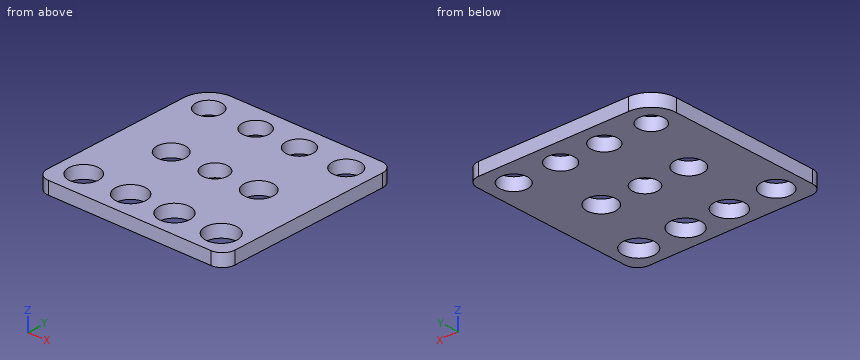
```python
from build123d import *

# Parameters (mm, degrees)
CROQUIS1_R              = 2.2
CROQUIS1_R_2            = 2.5
CROQUIS1_R_3            = 2.35
CROQUIS1_R_4            = 2.05
CROQUIS1_R_5            = 2.1
CROQUIS1_R_6            = 2.15
CROQUIS1_R_7            = 2.4
CROQUIS1_R_8            = 2.45
CROQUIS1_R_9            = 2.25
CROQUIS1_R_10           = 2.3
CROQUIS1_R_11           = 2
SALIENTE_EXTRUIR1_DEPTH = 2


with BuildPart() as part:
    # Croquis1 → Saliente-Extruir1 (new body)
    with BuildSketch(Plane.XY):
        with BuildLine():
            Line((-84.957262486, 47.717592446), (-60.957262486, 47.717592446))
            ThreePointArc((-60.957262486, 47.717592446), (-59.543048923, 47.131806009), (-58.957262486, 45.717592446))
            Line((-58.957262486, 45.717592446), (-58.957262486, 19.717592446))
            ThreePointArc((-58.957262486, 19.717592446), (-59.543048923, 18.303378884), (-60.957262486, 17.717592446))
            Line((-60.957262486, 17.717592446), (-86.957262486, 17.717592446))
            ThreePointArc((-86.957262486, 17.717592446), (-88.371476048, 18.303378884), (-88.957262486, 19.717592446))
            Line((-88.957262486, 19.717592446), (-88.957262486, 43.717592446))
            ThreePointArc((-88.957262486, 43.717592446), (-87.78568961, 46.546019571), (-84.957262486, 47.717592446))
        make_face()
        with Locations((-62.957262486, 43.717592446)):
            Circle(CROQUIS1_R, mode=Mode.SUBTRACT)
        with Locations((-62.957262486, 21.717592446)):
            Circle(CROQUIS1_R_2, mode=Mode.SUBTRACT)
        with Locations((-84.957262486, 21.717592446)):
            Circle(CROQUIS1_R_3, mode=Mode.SUBTRACT)
        with Locations((-84.957262486, 43.717592446)):
            Circle(CROQUIS1_R_4, mode=Mode.SUBTRACT)
        with Locations((-77.457263515, 43.721521604)):
            Circle(CROQUIS1_R_5, mode=Mode.SUBTRACT)
        with Locations((-70.457261138, 43.722088276)):
            Circle(CROQUIS1_R_6, mode=Mode.SUBTRACT)
        with Locations((-77.457263515, 21.721521604)):
            Circle(CROQUIS1_R_7, mode=Mode.SUBTRACT)
        with Locations((-70.457261138, 21.722088276)):
            Circle(CROQUIS1_R_8, mode=Mode.SUBTRACT)
        with Locations((-80.957262486, 32.717592446)):
            Circle(CROQUIS1_R_9, mode=Mode.SUBTRACT)
        with Locations((-66.957262486, 32.717592446)):
            Circle(CROQUIS1_R_10, mode=Mode.SUBTRACT)
        with Locations((-73.957262486, 32.717592446)):
            Circle(CROQUIS1_R_11, mode=Mode.SUBTRACT)
    extrude(amount=SALIENTE_EXTRUIR1_DEPTH)


solid = part.part
```
CAD build for the part. Positions are in the model's coordinates, mm. Round coordinates to 2 decimals unless told otherwise and drop trailing zeros. Write each loop counter-clockwise with the first axis right and the second up, starting at its lowest first coordinate (ties: lowest second). Pieces come first, ordered by that corner, then holes.
Item 1: Band-saw the part on C-C on z = 1.35. Give the number of separate pieces and of enclosed holes in the cut face, then the cut area to 3 significant figures.
Filled in:
separate pieces: 1
enclosed holes: 11
area: 718 mm2
Item 2: Band-saw the part on B-B on y = 22.5. Write the cut outline in (x, z).
Filled in:
outline: (-88.96, 0) - (-87.17, 0) - (-87.17, 2) - (-88.96, 2) - close; (-82.74, 0) - (-79.73, 0) - (-79.73, 2) - (-82.74, 2) - close; (-75.19, 0) - (-72.78, 0) - (-72.78, 2) - (-75.19, 2) - close; (-68.13, 0) - (-65.33, 0) - (-65.33, 2) - (-68.13, 2) - close; (-60.58, 0) - (-58.96, 0) - (-58.96, 2) - (-60.58, 2) - close
Item 3: Drop a flat-ended pin along its axis: pin 1 Ø3 at (x, y) = (-70.46, 21.72) entering from +Z. Give the stop position or say it passes through.
Filled in:
pin 1: passes through
Item 4: Band-saw the part on A-A on x = -86. Write the cut outline in (y, z).
Filled in:
outline: (17.72, 0) - (19.61, 0) - (19.61, 2) - (17.72, 2) - close; (23.82, 0) - (41.95, 0) - (41.95, 2) - (23.82, 2) - close; (45.48, 0) - (47.58, 0) - (47.58, 2) - (45.48, 2) - close
Item 5: Band-saw the part on D-D on x = -74. Write the cut outline in (y, z), then the cut area to 3 significant figures.
Filled in:
outline: (17.72, 0) - (30.72, 0) - (30.72, 2) - (17.72, 2) - close; (34.72, 0) - (47.72, 0) - (47.72, 2) - (34.72, 2) - close
area: 52.0 mm2
Item 6: Drill centre lines: L1, parallel to Y at x = -62, z = 1.2; L2, parallel to Y at x = -61, z = 1.2; L3, parallel to X at y = 33, z = 1.25. Where is each one in solid material? Low to high.
Filled in:
L1: y = 17.72 to 19.41, 24.03 to 41.74, 45.7 to 47.72
L2: y = 17.72 to 20.16, 23.27 to 42.71, 44.72 to 47.72
L3: x = -88.96 to -83.19, -78.73 to -75.94, -71.98 to -69.24, -64.67 to -58.96
